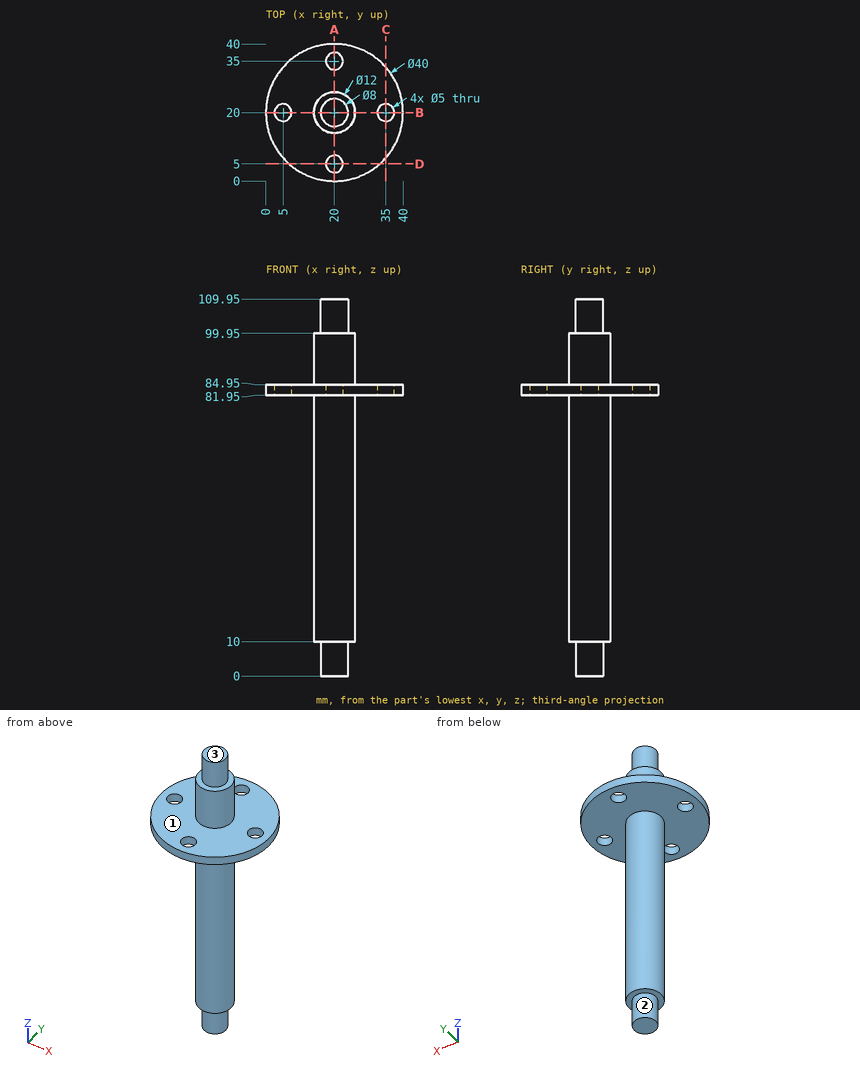
The drawing under review shows one solid part. Ordinate dimensions are in mm from its lowest x, y, z. A direction names the side the tool comes from. Coordinates: 2 decimals unless noted, no trailing zeros. Loops run counter-clockwise (first coordinate to the right, second up) from the corner with the lowest first, then second, coordinate; pieces in that order, holes last. Notation, with made-up numbers: (59.5, 52.25) -> (84.5, 52.25) arc R11 cw to (84.5, 72.25) -> close; hole circle Ø11 at (40.5, -4.75). An arc over 180 degrees is marked (long way). Answer as a JSON object with one key per item and string values.
Q1. Take a section at C-C on x = 35. Give the boundary of the cut face in (y, z), plus the area to 3 significant figures.
Answer block:
{"outline": "(6.77, 81.95) -> (17.5, 81.95) -> (17.5, 84.95) -> (6.77, 84.95) -> close; (22.5, 81.95) -> (33.23, 81.95) -> (33.23, 84.95) -> (22.5, 84.95) -> close", "area": "64.4 mm^2"}
Q2. To check wall thickness, follow L1, parallel to Y at x = 20, z = 84.25; L2, parallel to Z at x = 14.5, y = 38.5; L3, parallel to Y at x = 5, z = 83.9. State the ranges of each line that lie inside material, in increasing order.
Answer block:
{"L1": "y = 0 to 2.5, 7.5 to 32.5, 37.5 to 40", "L2": "z = 81.95 to 84.95", "L3": "y = 6.77 to 17.5, 22.5 to 33.23"}
Q3. Take a section at A-A on x = 20. Give the boundary of the cut face in (y, z).
Answer block:
{"outline": "(0, 81.95) -> (2.5, 81.95) -> (2.5, 84.95) -> (0, 84.95) -> close; (7.5, 81.95) -> (14, 81.95) -> (14, 10) -> (16, 10) -> (16, 0) -> (24, 0) -> (24, 10) -> (26, 10) -> (26, 81.95) -> (32.5, 81.95) -> (32.5, 84.95) -> (26, 84.95) -> (26, 99.95) -> (24, 99.95) -> (24, 109.95) -> (16, 109.95) -> (16, 99.95) -> (14, 99.95) -> (14, 84.95) -> (7.5, 84.95) -> close; (37.5, 81.95) -> (40, 81.95) -> (40, 84.95) -> (37.5, 84.95) -> close"}
Q4. Tool access review of the marked faces 1, 2 and 3: name each direction out of +Z, -Z, +X, -X, +Y, -Y from which nothing blocks a thin tool from reaching the whole face with its end or side.
Answer block:
{"face 1": "+Z", "face 2": "-Z", "face 3": "+Z, +X, -X, +Y, -Y"}
Q5. Clearance check with flat-ended pins moving along their axes: pin 1 Ø4 at (x, z) = (18.5, 34.5) entering from +Y; pin 2 Ø1 at (x, z) = (18.5, 42.5) entering from -Y; pin 3 Ø12 at (x, y) = (29, 30) entering from -Z; pin 4 Ø3.5 at (x, y) = (17, 21) entering from -Z. State where each tip first meets the part, or that it passes through.
Answer block:
{"pin 1": "stops at y = 26", "pin 2": "stops at y = 14.08", "pin 3": "stops at z = 81.95", "pin 4": "stops at z = 0"}
